CAD build for the part. Positions are in the model's coordinates, mm. A direction names the side the tool comes from. Round coordinates to 2 decimals unless told otherwise and drop trailing zeros. Write each loop counter-clockwise with the first axis right and the second up, starting at its lowest first coordinate (ties: lowest second). Pieces come first, ordered by that corner, then holes. Notation, with made-up numbers: (-15, -27.75) - (36, -27.75) arc R14 cw to (36, -15.75) - close; hole circle Ø5 at (24, 43). An arc over 180 degrees is marked (long way). Put each result on its own line as item: value. Start each with the question number.
Item 1: Pin check, flat tips, straight feed: pin 1 Ø0.8 at (y, z) = (2, -11.5) entering from +X (3 decimals); pin 2 Ø1.2 at (y, z) = (1, -12) entering from -X (3 decimals). Stop position of each tip, or through.
Item 2: 3-axis set-ups, long thin cutter, end or side, ignore diameter. For faces 1 (the flat face through (-11, 2, -18)), 2 (the flat face through (0, 2, -30)), 3 (the flat face through (-15, 2, -17)), 4 (the flat face through (18, 2, -10)): which of +Z, -Z, +X, -X, +Y, -Y reach the whole face in a straight line?
Item 3: Mould opens along X. For faces 5 (the flat face through (-14, 2, -12)), 6 (the flat face through (15, 2, -17)), 7 (the flat face through (10, 2, -15)) say: released by +X, released by -X, zero draft, split by the parting line, or undercut.
Item 4: Cut at A-A (z = -18). Give the cut face in (x, y) (3 decimals), and give its area (3 significant figures).
Item 5: Drill centre lines: line 1 (X direction, y = 2.5, z = -11) (3 decimals); line 2 (Z direction, x = 11.5, y = 2.4); line 3 (Z direction, x = -16, y = 0.3). Where is each one in solid material? Low to high. Write a range as from..to.
Item 6: Cut at B-B (x = 17.5). Give the cut face in (y, z) (3 decimals).
```python
from build123d import *

# Parameters (mm, degrees)
BOSS_EXTRUDE1_DEPTH = 3.175


with BuildPart() as part:
    # Sketch2 → Boss-Extrude1 (new body)
    with BuildSketch(Plane(origin=(0, 0, 0), x_dir=(1, 0, 0), z_dir=(0, 1, 0))):
        Polygon((20, 20), (20, 30), (0, 30), (0, 0), (20, 0), (20, 10), (16.825, 10), (16.825, 13), (14, 13), (14, 10.5), (11, 10.5), (11, 13), (10, 13), (10, 17), (11, 17), (11, 19.5), (14, 19.5), (14, 17), (16.825, 17), (16.825, 20), align=None)
    boss_extrude1 = extrude(amount=BOSS_EXTRUDE1_DEPTH)

    # Mirror1: Boss-Extrude1 across plane
    add(boss_extrude1.mirror(Plane(origin=(0, 3.175, 0), x_dir=(0, 0, 1), z_dir=(1, 0, 0))))


solid = part.part
```
Output values:
1. pin 1: x = 16.825
1. pin 2: x = -16.825
2. face 1: +Y, -Y
2. face 2: -Z, +X, -X, +Y, -Y
2. face 3: -X, +Y, -Y
2. face 4: +X, +Y, -Y
3. face 5: undercut
3. face 6: zero draft
3. face 7: released by +X
4. outline: (-16.825, 0) - (-14, 0) - (-14, 3.175) - (-16.825, 3.175) - close; (-11, 0) - (11, 0) - (11, 3.175) - (-11, 3.175) - close; (14, 0) - (16.825, 0) - (16.825, 3.175) - (14, 3.175) - close
4. area: 87.8 mm2
5. line 1: -16.825..-14, -11..11, 14..16.825
5. line 2: -30..-19.5, -10.5..0
5. line 3: -30..-17, -13..0
6. outline: (0, -30) - (3.175, -30) - (3.175, -20) - (0, -20) - close; (0, -10) - (3.175, -10) - (3.175, 0) - (0, 0) - close
